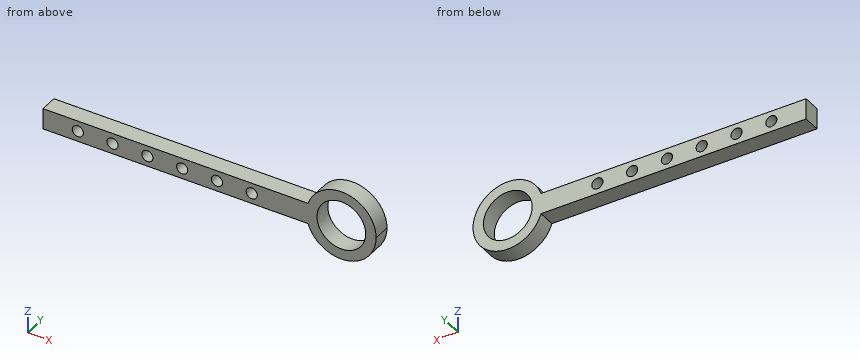
```python
from build123d import *

# Parameters (mm, degrees)
SKETCH1_R           = 7
BOSS_EXTRUDE1_DEPTH = 5


with BuildPart() as part:
    # Sketch1 → Boss-Extrude1 (new body)
    # profile 1 of 7: a face of its own
    with BuildSketch(Plane(origin=(0, 0, 0), x_dir=(1, 0, 0), z_dir=(0, 1, 0))):
        with BuildLine():
            Line((76.2, 3), (76.2, 0))
            ThreePointArc((76.2, 0), (87.256969007, -6.884177258), (95.739392014, 3))
            ThreePointArc((95.739392014, 3), (87.256969007, 12.884177258), (76.2, 6))
            Line((76.2, 6), (76.2, 3))
        make_face()
        with Locations(Location((85.739392014, 3, 0), (0, 0, 270))):
            Circle(SKETCH1_R, mode=Mode.SUBTRACT)
    # profile 2 of 7: a face of its own
    with BuildSketch(Plane(origin=(0, 0, 0), x_dir=(1, 0, 0), z_dir=(0, 1, 0))):
        with BuildLine():
            ThreePointArc((75.739392014, 3), (75.855214756, 1.482423007), (76.2, 0))
            Line((76.2, 0), (76.2, 3))
            Line((76.2, 3), (75.739392014, 3))
        make_face()
    # profile 3 of 7: a face of its own
    with BuildSketch(Plane(origin=(0, 0, 0), x_dir=(1, 0, 0), z_dir=(0, 1, 0))):
        with BuildLine():
            Line((76.2, 3), (76.2, 6))
            ThreePointArc((76.2, 6), (75.855214756, 4.517576993), (75.739392014, 3))
            Line((75.739392014, 3), (76.2, 3))
        make_face()
    # profile 4 of 7: a face of its own
    with BuildSketch(Plane(origin=(0, 0, 0), x_dir=(1, 0, 0), z_dir=(0, 1, 0))):
        with BuildLine():
            ThreePointArc((75.739392014, 3), (75.855214756, 1.482423007), (76.2, 0))
            Line((76.2, 0), (76.2, 3))
            Line((76.2, 3), (75.739392014, 3))
        make_face()
    # profile 5 of 7: a face of its own
    with BuildSketch(Plane(origin=(0, 0, 0), x_dir=(1, 0, 0), z_dir=(0, 1, 0))):
        with BuildLine():
            Line((76.2, 3), (76.2, 6))
            ThreePointArc((76.2, 6), (75.855214756, 4.517576993), (75.739392014, 3))
            Line((75.739392014, 3), (76.2, 3))
        make_face()
    # profile 6 of 7: a face of its own
    with BuildSketch(Plane(origin=(0, 0, 0), x_dir=(1, 0, 0), z_dir=(0, 1, 0))):
        with BuildLine():
            Line((8.4, 3), (0, 3))
            Line((0, 3), (0, 0))
            Line((0, 0), (76.2, 0))
            ThreePointArc((76.2, 0), (75.855214756, 1.482423007), (75.739392014, 3))
            Line((75.739392014, 3), (61.6, 3))
            ThreePointArc((61.6, 3), (60, 1.4), (58.4, 3))
            Line((58.4, 3), (51.6, 3))
            ThreePointArc((51.6, 3), (50, 1.4), (48.4, 3))
            Line((48.4, 3), (41.6, 3))
            ThreePointArc((41.6, 3), (40, 1.4), (38.4, 3))
            Line((38.4, 3), (31.6, 3))
            ThreePointArc((31.6, 3), (30, 1.4), (28.4, 3))
            Line((28.4, 3), (21.6, 3))
            ThreePointArc((21.6, 3), (20, 1.4), (18.4, 3))
            Line((18.4, 3), (11.6, 3))
            ThreePointArc((11.6, 3), (10, 1.4), (8.4, 3))
        make_face()
    # profile 7 of 7: a face of its own
    with BuildSketch(Plane(origin=(0, 0, 0), x_dir=(1, 0, 0), z_dir=(0, 1, 0))):
        with BuildLine():
            Line((0, 6), (0, 3))
            Line((0, 3), (8.4, 3))
            ThreePointArc((8.4, 3), (10, 4.6), (11.6, 3))
            Line((11.6, 3), (18.4, 3))
            ThreePointArc((18.4, 3), (20, 4.6), (21.6, 3))
            Line((21.6, 3), (28.4, 3))
            ThreePointArc((28.4, 3), (30, 4.6), (31.6, 3))
            Line((31.6, 3), (38.4, 3))
            ThreePointArc((38.4, 3), (40, 4.6), (41.6, 3))
            Line((41.6, 3), (48.4, 3))
            ThreePointArc((48.4, 3), (50, 4.6), (51.6, 3))
            Line((51.6, 3), (58.4, 3))
            ThreePointArc((58.4, 3), (60, 4.6), (61.6, 3))
            Line((61.6, 3), (75.739392014, 3))
            ThreePointArc((75.739392014, 3), (75.855214756, 4.517576993), (76.2, 6))
            Line((76.2, 6), (0, 6))
        make_face()
    extrude(amount=BOSS_EXTRUDE1_DEPTH)


solid = part.part
```
Geometry check sheet. Reference: the model listing, model coordinates, mm. Coordinates: 2 decimals unless noted, no trailing zeros. Order: outer loops, then holes, each group sorted by start corner. A loop starts at its lowest first (then second) coordinate and runs counter-clockwise, first axis right, second up. Notation, with made-up numbers: M 53.25,-15 L 66.25,-15 A11 cw 66.25,-7 Z; hole C 67.5,-10 d6. An arc over 180 degrees is marked long. Answer as a JSON object with one key per item and string values.
Q1. Scan lines: line 1 (Z direction, x = 30, y = 3.5); line 2 (Z direction, x = 48, y = 1.4); line 3 (X direction, y = 1.6, z = -0.5). Record each from-to range of solid material in increasing order.
Results are:
{"line 1": "z = -6 to -4.6, -1.4 to 0", "line 2": "z = -6 to 0", "line 3": "x = 0 to 79.2, 92.28 to 95.42"}
Q2. Cross-section at A-A on x = 50. Record the cut outline in (y, z), and give its area (3 significant figures).
Results are:
{"outline": "M 0,-6 L 5,-6 L 5,-4.6 L 0,-4.6 Z; M 0,-1.4 L 5,-1.4 L 5,0 L 0,0 Z", "area": "14.0 mm²"}
Q3. Depth check by flat-ended pin: pin 1 Ø1.5 at (y, z) = (0.5, 1) entering from -X; pin 2 Ø3 at (y, z) = (1, -9.5) entering from -X; pin 3 Ø1.5 at (x, y) = (52.5, 1.5) entering from +Z. Enter the tip coordinate at first touch or a pass-through.
Results are:
{"pin 1": "stops at x = 76.28", "pin 2": "stops at x = 77.08", "pin 3": "stops at z = 0"}
Q4. Cross-section at B-B on y = 3.3. Record the cut outline in (x, z).
Results are:
{"outline": "M 0,-6 L 76.2,-6 A10 ccw long 76.2,0 L 0,0 Z; hole C 10,-3 d3.2; hole C 20,-3 d3.2; hole C 30,-3 d3.2; hole C 40,-3 d3.2; hole C 50,-3 d3.2; hole C 60,-3 d3.2; hole C 85.74,-3 d14"}
Q5. Cross-section at C-C on z = 2.5. Record the cut outline in (x, y).
Results are:
{"outline": "M 77.39,0 L 81.41,0 L 81.41,5 L 77.39,5 Z; M 90.07,0 L 94.09,0 L 94.09,5 L 90.07,5 Z"}
